Build history of the part. All positions in model axes, mm. A direction names the side the tool comes from. Coordinates: 2 decimals unless noted, no trailing zeros. Loops run counter-clockwise (first coordinate to the right, second up) from the corner with the lowest first, then second, coordinate; pieces in that order, holes last.
Item 1: Cut at B-B (y = -58.5). List the corners of the cut face in (x, z).
Item 2: Drill centre lines: line 1 along X through (y, z) = (-61.5, 1.5); line 2 along Y through (x, z) = (-13.25, 13.5). Where is each one in solid material? Low to high.
Item 3: Cut at A-A (z = 12.5). List the corners of the cut face in (x, y).
Item 4: Cut at C-C (x = 11). List the corners of the cut face in (y, z).
Item 5: 3-axis set-ups, long thin cutter, end or side, ignore diameter. For faces 1 (the face through (-10, -50, 15)), 2 (the face through (10, -50, 15)), 3 (the face through (0, 25, 15)): which of +Z, -Z, +X, -X, +Y, -Y reach the whole face in a straight line?
Item 6: Flat gauge pins, fed straight in: pin 1 (4 mm diameter, centred on y = -50, z = 17, fed in from +X); pin 2 (1.5 mm diameter, centred on x = -12, z = 18, fed in from -Y); pin 3 (4 mm diameter, centred on x = 2.5, y = -19.5, fed in from -Z); pin 4 (12 mm diameter, centred on y = -44, z = 25.5, fed in from -X). Where does each tip first touch, or does it go through?
Autodesk Inventor part; units mm, degrees
sketch "Sketch1" plane through (0, 0, 0) normal (0, 0, 1) x (1, 0, 0)
  line L0 (-15, 25) -> (15, 25)
  line L1 (15, 25) -> (15, -25)
  line L2 (15, -25) -> (-15, -25)
  line L3 (-15, -25) -> (-15, 25)
  point P0 (0, 0)
  point P1 (0, 25)
  point P2 (-15, 0)
  dimension "d0" = 50
  dimension "d1" = 30
extrude "Extrusion1" add sketch "Sketch1" along normal blind 30
sketch "Sketch2" plane through (0, 0, 30) normal (0, 0, 1) x (1, 0, 0)
  line L0 (-15, -25) -> (15, -25)
  line L1 (-10, -25) -> (10, -25)
  line L2 (10, -25) -> (10, -75)
  line L3 (10, -75) -> (-10, -75)
  line L4 (-10, -75) -> (-10, -25)
  point P0 (0, 0)
  point P1 (0, -25)
  point P2 (0, -25)
  dimension "d4" = 20
  dimension "d5" = 50
extrude "Extrusion2" add sketch "Sketch2" against normal blind 30
properties part number "Actuator"
Filled sheet:
1. outline: (-10, 0) - (10, 0) - (10, 30) - (-10, 30) - close
2. line 1: x = -10 to 10
2. line 2: y = -25 to 25
3. outline: (-15, -25) - (-10, -25) - (-10, -75) - (10, -75) - (10, -25) - (15, -25) - (15, 25) - (-15, 25) - close
4. outline: (-25, 0) - (25, 0) - (25, 30) - (-25, 30) - close
5. face 1: +Z, -Z, -X, -Y
5. face 2: +Z, -Z, +X, -Y
5. face 3: +Z, -Z, +X, -X, +Y
6. pin 1: stops at x = 10
6. pin 2: stops at y = -25
6. pin 3: stops at z = 0
6. pin 4: stops at x = -10
